```python
from build123d import *

# Parameters (mm, degrees)
F0_W     = 86.5
F0_H     = 60.5
F1_DEPTH = 4
F3_DEPTH = 59
F4_R     = 1.75
F5_DEPTH = 63.001


with BuildPart() as f1:
    # F0 (on Top) → F1 (new body)
    with BuildSketch(Plane.XY):
        Rectangle(F0_W, F0_H)
    extrude(amount=F1_DEPTH)

    # F2 (on face) → F3 (join)
    with BuildSketch(Plane.XY.offset(4)):
        Polygon((37.25, -24.75), (37.25, 25.25), (-37.25, 25.25), (-37.25, 7.3957513111), (-37.25, -24.75), align=None)
        Polygon((-32.25, 2.1042486889), (-32.25, 7.3957513111), (-32.25, 20.25), (32.25, 20.25), (32.25, 7.3957513111), (32.25, 2.1042486889), (32.25, -19.75), (-32.25, -19.75), align=None, mode=Mode.SUBTRACT)
        with BuildLine():
            Line((26.1275010008, 7.25), (-26.1275010008, 7.25))
            ThreePointArc((-26.1275010008, 7.25), (-29.154803559, 8.7488670443), (-32.25, 7.3957513111))
            Line((-32.25, 7.3957513111), (-32.25, 2.1042486889))
            ThreePointArc((-32.25, 2.1042486889), (-29.154803559, 0.7511329557), (-26.1275010008, 2.25))
            Line((-26.1275010008, 2.25), (26.1275010008, 2.25))
            ThreePointArc((26.1275010008, 2.25), (29.154803559, 0.7511329557), (32.25, 2.1042486889))
            Line((32.25, 2.1042486889), (32.25, 7.3957513111))
            ThreePointArc((32.25, 7.3957513111), (29.154803559, 8.7488670443), (26.1275010008, 7.25))
        make_face()
    extrude(amount=F3_DEPTH)

    # F4 (on face) → F5 (cut, through all)
    with BuildSketch(Plane.XY.offset(63)):
        with Locations((-29.25, 4.75)):
            Circle(F4_R)
        with Locations((29.25, 4.75)):
            Circle(F4_R)
    extrude(amount=-F5_DEPTH, mode=Mode.SUBTRACT)


solid = f1.part
```
Geometry check sheet. Reference: the model listing, model coordinates, mm. A direction names the side the tool comes from. Give positions to 0.01 mm unless a question says otherwise; leave off trailing zeros. Write each loop counter-clockwise with the first axis right and the second up, starting at its lowest first coordinate (ties: lowest second). Pieces come first, ordered by that corner, then holes. Notation, with made-up numbers: (-15, 51.5) - (11, 51.5) arc R21 ccw to (11, 78.5) - close; hole circle Ø5 at (67, 16.25). An arc over 180 degrees is marked (long way). Use a Markdown table: item, result.
Q1. Set-up check for faces 4 (the face through (0, 14, 4)), 5 (the face through (-1, -24.75, 33)), 6 (the face through (-43.25, 0, 2)): record each of +Z, -Z, +X, -X, +Y, -Y from which the full face is reachable in a straight line by a thin tool's end or side.
Computed:
| item | result |
|---|---|
| face 4 | +Z |
| face 5 | +Z, +X, -X, -Y |
| face 6 | +Z, -Z, -X, +Y, -Y |
Q2. Go/stop test with flat-tipped pins: P1, Ø17.5, axis at y = -7.5, z = 21.5, coming from the +X side; P2, Ø11, axis at y = -13, z = 45, coming from the -X side; P3, Ø10, axis at x = -29, z = 10, coming from the -Y side. Record where each tip stops, or that it passes through.
Computed:
| item | result |
|---|---|
| P1 | stops at x = 37.25 |
| P2 | stops at x = -37.25 |
| P3 | stops at y = -24.75 |
Q3. Section check C-C, the plane x = 29.25. Enter the section's corners in (y, z), then the cut area to 3 significant figures.
Computed:
| item | result |
|---|---|
| outline | (-30.25, 0) - (3, 0) - (3, 63) - (0.75, 63) - (0.75, 4) - (-19.75, 4) - (-19.75, 63) - (-24.75, 63) - (-24.75, 4) - (-30.25, 4) - close; (6.5, 0) - (30.25, 0) - (30.25, 4) - (25.25, 4) - (25.25, 63) - (20.25, 63) - (20.25, 4) - (8.75, 4) - (8.75, 63) - (6.5, 63) - close |
| area | 1,080 mm² |
Q4. Section check B-B, the plane z = 59.5. Enter the section's corners in (x, y), then the cut area to 3 significant figures.
Computed:
| item | result |
|---|---|
| outline | (-37.25, -24.75) - (37.25, -24.75) - (37.25, 25.25) - (-37.25, 25.25) - close; hole (-32.25, -19.75) - (32.25, -19.75) - (32.25, 2.1) arc R4 cw to (26.13, 2.25) - (-26.13, 2.25) arc R4 cw to (-32.25, 2.1) - close; hole (-32.25, 7.4) arc R4 cw to (-26.13, 7.25) - (26.13, 7.25) arc R4 cw to (32.25, 7.4) - (32.25, 20.25) - (-32.25, 20.25) - close; hole circle Ø3.5 at (-29.25, 4.75); hole circle Ø3.5 at (29.25, 4.75) |
| area | 1,470 mm² |
Q5. Draft check along X on faces 1 (the face through (37.25, 0, 33)), 2 (the face through (32.25, 14, 33)), 3 (the face through (-1, -26, 4)). Enter one of: pulls with the +X half, pulls with the -X half, needs draft (parallel to the pull), parting line crosses it, or undercut.
Computed:
| item | result |
|---|---|
| face 1 | pulls with the +X half |
| face 2 | undercut |
| face 3 | needs draft |
Q6. Section check A-A, the plane y = 4.75. Enter the section's corners in (x, z), then the cut area to 3 significant figures.
Computed:
| item | result |
|---|---|
| outline | (-43.25, 0) - (-31, 0) - (-31, 63) - (-37.25, 63) - (-37.25, 4) - (-43.25, 4) - close; (-27.5, 0) - (27.5, 0) - (27.5, 63) - (-27.5, 63) - close; (31, 0) - (43.25, 0) - (43.25, 4) - (37.25, 4) - (37.25, 63) - (31, 63) - close |
| area | 4,300 mm² |
Q7. Thickness scan on L1, parallel to Y at x = 29, z = 41; L2, parallel to Y at x = -25.5, z = 32.5; L3, parallel to X at y = -18, z = 33. Record the ranges inside material, lowest first. Write a range as [from, to].
Computed:
| item | result |
|---|---|
| L1 | y = [-24.75, -19.75], [0.76, 3.02], [6.48, 8.74], [20.25, 25.25] |
| L2 | y = [-24.75, -19.75], [2.25, 7.25], [20.25, 25.25] |
| L3 | x = [-37.25, -32.25], [32.25, 37.25] |
Q8. Section check D-D, the plane x = -24. Enter the section's corners in (y, z).
Computed:
| item | result |
|---|---|
| outline | (-30.25, 0) - (30.25, 0) - (30.25, 4) - (25.25, 4) - (25.25, 63) - (20.25, 63) - (20.25, 4) - (7.25, 4) - (7.25, 63) - (2.25, 63) - (2.25, 4) - (-19.75, 4) - (-19.75, 63) - (-24.75, 63) - (-24.75, 4) - (-30.25, 4) - close |
